from build123d import *

# Parameters (mm, degrees)
SKETCH2_R           = 12.5
SKETCH2_R_2         = 8
SKETCH2_R_3         = 13
BOSS_EXTRUDE1_DEPTH = 5
CUT_EXTRUDE1_DEPTH  = 3


with BuildPart() as part:
    # Sketch2 → Boss-Extrude1 (new, symmetric)
    # profile 1 of 3: a face of its own
    with BuildSketch(Plane.XY):
        with Locations((0, 130)):
            Circle(SKETCH2_R)
        with Locations((0, 130)):
            Circle(SKETCH2_R_2, mode=Mode.SUBTRACT)
    # profile 2 of 3: a face of its own
    with BuildSketch(Plane.XY):
        with BuildLine():
            Line((-12.5, 130), (-22.235294118, 3.441176471))
            ThreePointArc((-22.235294118, 3.441176471), (0, 22.5), (22.235294118, 3.441176471))
            Line((22.235294118, 3.441176471), (12.5, 130))
            ThreePointArc((12.5, 130), (0, 117.5), (-12.5, 130))
        make_face()
    # profile 3 of 3: a face of its own
    with BuildSketch(Plane.XY):
        with BuildLine():
            Line((-22.235294118, 3.441176471), (-22.5, 0))
            ThreePointArc((-22.5, 0), (0, -22.5), (22.5, 0))
            Line((22.5, 0), (22.235294118, 3.441176471))
            ThreePointArc((22.235294118, 3.441176471), (0, 22.5), (-22.235294118, 3.441176471))
        make_face()
        Circle(SKETCH2_R_3, mode=Mode.SUBTRACT)
    extrude(amount=BOSS_EXTRUDE1_DEPTH, both=True)

    # Sketch3 → Cut-Extrude1 (cut)
    with BuildSketch(Plane.XY.offset(5)):
        with BuildLine():
            Line((-8.257578004, 119.959461892), (-17.038818827, 5.803331197))
            ThreePointArc((-17.038818827, 5.803331197), (0, 18), (17.038818827, 5.803331197))
            Line((17.038818827, 5.803331197), (8.257578004, 119.959461892))
            ThreePointArc((8.257578004, 119.959461892), (0, 117), (-8.257578004, 119.959461892))
        make_face()
    cut_extrude1 = extrude(amount=-CUT_EXTRUDE1_DEPTH, mode=Mode.SUBTRACT)

    # Mirror1: Cut-Extrude1 across plane
    add(cut_extrude1.mirror(Plane.XY), mode=Mode.SUBTRACT)


solid = part.part
Here's how the part is built. I have some questions about the finished solid (model axes, mm). A direction names the side the tool comes from. Give positions to 0.01 mm unless a question says otherwise; leave off trailing zeros. Order: outer loops, then holes, each group sorted by start corner. A loop starts at its lowest first (then second) coordinate and runs counter-clockwise, first axis right, second up. Notation, with made-up numbers: (11, 22.5) -> (65, 22.5) arc R26 cw to (65, 49.5) -> close; hole circle Ø3 at (43, 36). An arc over 180 degrees is marked (long way). Use a Markdown table: item, result. Add a question column.
Item 1: I need wall thicknesses on line 1 (Y direction, x = 0, z = 2.45); line 2 (Y direction, x = 0, z = -1.95); line 3 (Y direction, x = -5, z = -4) (3 decimals). Which ranges of each line are inside material? Lowest first, please.
Item 2: If we mould it in two halves opening along X, with no side actions, what happens to faces 1 (the face through (15, 48, 5)), 2 (the face through (0, 64, 2)), 3 (the face through (-0.495, -22.495, 0.07))? For each: pulls with the +X half, pulls with the -X half, needs draft (parallel to the pull), parting line crosses it, or undercut.
Item 3: Will these pins go through, and if not, where does the flat tip stop? pin 1 (17 mm diameter, centred on x = 3, y = 36, fed in from -Z); pin 2 (1.5 mm diameter, centred on y = 13, z = -1, fed in from +X); pin 3 (4 mm diameter, centred on x = -7, z = -2, fed in from -Y).
Item 4: Imagine slicing it at C-C on y = 87.5. Please give me the cut outline in (x, z).
Item 5: Imagine slicing it at A-A on y = 127.5. Please give me the cut outline in (x, z).
Item 6: Imagine slicing it at B-B on x = 0. Please give me the cut outline in (y, z), plus the area to 3 significant figures.
Item 7: For faces 4 (the face through (-12.587, 63.68, 3.521)), 5 (the face through (0, 64, -2)), 6 (the face through (15, 48, -5)), which set-ups out of +Z, -Z, +X, -X, +Y, -Y let a thin tool reach every point of the face, with its end or its side?
Item 8: Imagine slicing it at D-D on x = 14.5. Please give me the cut outline in (y, z), plus the area to 3 significant figures.
Data:
| question | item | result |
|---|---|---|
| 1 | line 1 | y = -22.5 to -13, 13 to 18, 117 to 122, 138 to 142.5 |
| 1 | line 2 | y = -22.5 to -13, 13 to 122, 138 to 142.5 |
| 1 | line 3 | y = -21.937 to -12, 12 to 17.292, 118 to 123.755, 136.245 to 141.456 |
| 2 | face 1 | needs draft |
| 2 | face 2 | undercut |
| 2 | face 3 | parting line crosses it |
| 3 | pin 1 | stops at z = -2 |
| 3 | pin 2 | stops at x = 21.56 |
| 3 | pin 3 | stops at y = -21.94 |
| 4 | outline | (-15.77, -5) -> (-10.75, -5) -> (-10.75, -2) -> (10.75, -2) -> (10.75, -5) -> (15.77, -5) -> (15.77, 5) -> (10.75, 5) -> (10.75, 2) -> (-10.75, 2) -> (-10.75, 5) -> (-15.77, 5) -> close |
| 5 | outline | (-12.69, -5) -> (-7.6, -5) -> (-7.6, 5) -> (-12.69, 5) -> close; (7.6, -5) -> (12.69, -5) -> (12.69, 5) -> (7.6, 5) -> close |
| 6 | outline | (-22.5, -5) -> (-13, -5) -> (-13, 5) -> (-22.5, 5) -> close; (13, -5) -> (18, -5) -> (18, -2) -> (117, -2) -> (117, -5) -> (122, -5) -> (122, 5) -> (117, 5) -> (117, 2) -> (18, 2) -> (18, 5) -> (13, 5) -> close; (138, -5) -> (142.5, -5) -> (142.5, 5) -> (138, 5) -> close |
| 6 | area | 636 mm² |
| 7 | face 4 | +Z |
| 7 | face 5 | -Z |
| 7 | face 6 | -Z, +X, -X, +Y, -Y |
| 8 | outline | (-17.2, -5) -> (10.67, -5) -> (10.67, -2) -> (38.81, -2) -> (38.81, -5) -> (104, -5) -> (104, 5) -> (38.81, 5) -> (38.81, 2) -> (10.67, 2) -> (10.67, 5) -> (-17.2, 5) -> close |
| 8 | area | 1,040 mm² |
